from build123d import *

# Parameters (mm, degrees)
F1_DEPTH = 1
F2_R     = 2
F3_DEPTH = 2
F5_DEPTH = 1
F8_DEPTH = 8


with BuildPart() as f1:
    # F0 (on Top) → F1 (new body)
    with BuildSketch(Plane.XY):
        Polygon((0, -8), (0, 0), (-12, 0), (-12, -2), (-8, -8), align=None)
        Polygon((-12, 0), (0, 0), (0, 8), (-8, 8), (-12, 2), align=None)
    extrude(amount=F1_DEPTH)

    # F2 (on face) → F3 (join)
    with BuildSketch(Plane.XY.offset(1)):
        with Locations((-4, 4)):
            Circle(F2_R)
        with Locations((-4, -4)):
            Circle(F2_R)
    extrude(amount=F3_DEPTH)


with BuildPart() as f5:
    # F4 (on face) → F5 (new body)
    with BuildSketch(Plane.XY.offset(1)):
        Polygon((-8, 6.197224), (-8, 8), (-12, 2), (-12, -2), (-8, -8), (-8, -6.197224), (-11, -1.697224), (-11, 1.697224), align=None)
    extrude(amount=F5_DEPTH)


with BuildPart() as f1_1:
    add(f1.part)

    # F6: union F5
    add(f5.part)

    # F7 (on face) → F8 (join)
    with BuildSketch(Plane(origin=(-12, 0, 0), x_dir=(0, -1, 0), z_dir=(-1, 0, 0))):
        with BuildLine():
            ThreePointArc((0, 0), (0.707107, 0.292893), (1, 1))
            ThreePointArc((1, 1), (0.707107, 1.707107), (0, 2))
            ThreePointArc((0, 2), (-1, 1), (0, 0))
        make_face()
    extrude(amount=F8_DEPTH)

    # F9: F1 across face


with BuildPart() as f1_2:
    add(f1_1.part)
    add(f1_1.part.mirror(Plane(origin=(0, 0, 0.5), x_dir=(0, 1, 0), z_dir=(1, 0, 0))))


solid = f1_2.part
Geometry: final body of the model. Coordinates: model frame, mm. A direction names the side the tool comes from. Coordinates: 2 decimals unless noted, no trailing zeros. Order: outer loops, then holes, each group sorted by start corner. A loop starts at its lowest first (then second) coordinate and runs counter-clockwise, first axis right, second up. Notation, with made-up numbers: (-5, -25.5) - (39, -25.5) arc R13 ccw to (39, -8.5) - close; hole circle Ø1 at (-37.5, 23). An arc over 180 degrees is marked (long way). Use one line per item in the form item = value.
1) Section B-B (y = -3). Return loops of the section in (x, z).
Solutions:
outline = (-11.33, 0) - (11.33, 0) - (11.33, 2) - (10.13, 2) - (10.13, 1) - (5.73, 1) - (5.73, 3) - (2.27, 3) - (2.27, 1) - (-2.27, 1) - (-2.27, 3) - (-5.73, 3) - (-5.73, 1) - (-10.13, 1) - (-10.13, 2) - (-11.33, 2) - close
2) Section C-C (z = 2.45). Return loops of the section in (x, y), then the cut area to 3 significant figures.
Solutions:
outline = circle Ø4 at (-4, -4); circle Ø4 at (-4, 4); circle Ø4 at (4, -4); circle Ø4 at (4, 4)
area = 50.3 mm^2
3) Ray query, L1, parallel to X at y = 0.75, z = 1.4; L2, parallel to X at y = 3.75, z = 1.6; L3, parallel to Z at x = 6, y = 1.5. Return the intervals inside material, ascending.
Solutions:
L1 = -20 to -11, 11 to 20
L2 = -10.83 to -9.63, -5.98 to -2.02, 2.02 to 5.98, 9.63 to 10.83
L3 = 0 to 1
4) Set-up query: faces 1 (the face through (8, -7.1, 1.5)), 2 (the face through (-12, -1.4, 1)), 3 (the face through (0, 0, 1)), 4 (the face through (-11.2, 0, 2)). Return all of +Z, -Z, +X, -X, +Y, -Y with unobstructed straight access to the full face (end or side cutting, diameter ignored); none if empty.
Solutions:
face_1 = +Z, +Y, -Y
face_2 = -X, -Y
face_3 = +Z
face_4 = +Z, -X, +Y, -Y
5) Section A-A (x = 4). Return loops of the section in (y, z).
Solutions:
outline = (-8, 0) - (8, 0) - (8, 1) - (6, 1) - (6, 3) - (2, 3) - (2, 1) - (-2, 1) - (-2, 3) - (-6, 3) - (-6, 1) - (-8, 1) - close
6) Section D-D (x = 13.5). Return loops of the section in (y, z).
Solutions:
outline = (-1, 1) arc R1 ccw (long way) to (0, 2) arc R1 ccw to start
7) Pin query (flat end, axial travel): pin 1 (0.8 mm diameter, centred on y = -7, z = 1.5, fed in from +X); pin 2 (1.2 mm diameter, centred on x = -9.5, y = 2, fed in from +Z); pin 3 (1.1 mm diameter, centred on y = 7, z = 1.5, fed in from -X). Return the tip coordinate at first contact, or that it passes through.
Solutions:
pin_1 = 8.93
pin_2 = 1
pin_3 = -9.03
